Autodesk Inventor part; units mm, degrees
ref_plane "Work Plane1" through (36.2204, 0, -3.175) normal (1, 0, 0) x (0, 1, 0)
ref_plane "XZ Plane" through (0, 0, 0) normal (0, 1, 0) x (-1, 0, 0)
ref_plane "XY Plane" through (0, 0, 0) normal (0, 0, 1) x (1, 0, 0)
sketch "Sketch1" plane through (0, 0, 0) normal (0, 1, 0) x (-1, 0, 0)
  line L0 (-33.0454, 0) -> (0, 0)
  line L1 (0, 0) -> (0, 5.08)
  line L2 (0, 5.08) -> (3.175, 5.08)
  line L3 (-33.0454, 0) -> (-33.0454, -3.175)
  line L4 (-33.0454, -3.175) -> (-36.2204, -3.175)
  dimension "d1" = 33.0454
  dimension "d6" = 5.08
  dimension "d7" = 3.175
  dimension "d8" = 3.175
  dimension "d9" = 3.175
ref_plane "Work Plane1" through (36.2204, 0, -3.175) normal (1, 0, 0) x (0, 1, 0)
sketch "Sketch2" plane through (36.2204, 0, -3.175) normal (1, 0, 0) x (0, 1, 0)
  circle A0 centre (0, 0) radius 0.8
  point P0 (0, 3.175)
  dimension "d10" = 1.6
sweep "Sweep1" add profiles "Sketch2" path "Sketch1"
properties part number "foreDivePlanesLinkage" material "Stainless Steel"
Here's how the part is built. I have some questions about the finished solid (model axes, mm). A direction names the side the tool comes from. Give positions to 0.01 mm unless a question says otherwise; leave off trailing zeros. Write each loop counter-clockwise with the first axis right and the second up, starting at its lowest first coordinate (ties: lowest second). Pieces come first, ordered by that corner, then holes. Notation, with made-up numbers: (39.5, -38) -> (98.5, -38) arc R32 cw to (98.5, -5) -> close; hole circle Ø8 at (-21.5, 15). An arc over 180 degrees is marked (long way). Use one line per item in the form item = value.
1) If I drill on L1, parallel to X at y = 0.05, z = -2.5; L2, parallel to Z at x = 22.5, y = 0.1; L3, parallel to X at y = 0, z = -0.25, over which ranges is the centre line in solid material (lowest first)? Write a range as [from, to].
Verdict:
L1 = [32.25, 36.22]
L2 = [-0.79, 0.79]
L3 = [-0.8, 33.85]
2) I'm going to push a flat-ended pin straight in: pin 1 (2 mm diameter, centred on x = 6.5, z = -1, fed in from +Y). Where does the tip first touch, or does it pass through?
Verdict:
pin_1 = 0.8
3) On a 3-axis mill with a long thin cutter (end or side, diameter ignored), from which of +Z, -Z, +X, -X, +Y, -Y can I reach the whole of each face in a straight line? I mean faces 1 (the face through (16.28, -0.63, 0.49)), 2 (the face through (-1.66, -0.17, 5.86)), 3 (the face through (-3.175, 0, 5)), 4 (the face through (36.22, 0, -3)), 5 (the face through (34.65, -0.1, -3.97)). Say none if no direction works.
Verdict:
face_1 = none
face_2 = -X
face_3 = +Z, -Z, -X, +Y, -Y
face_4 = +Z, -Z, +X, +Y, -Y
face_5 = +X
4) Suppose I cut it at A-A (y = 0). Please give me the cut outline in (x, z) (3 decimals), and give its area (3 significant figures).
Verdict:
outline = (-3.175, 4.28) -> (-0.8, 4.28) -> (-0.8, -0.8) -> (32.245, -0.8) -> (32.245, -3.975) -> (36.22, -3.975) -> (36.22, -2.375) -> (33.845, -2.375) -> (33.845, 0.8) -> (0.8, 0.8) -> (0.8, 5.88) -> (-3.175, 5.88) -> close
area = 76.2 mm2
5) Suppose I cut it at B-B (z = 2). Please give me the cut outline in (x, y), and give its area (3 significant figures).
Verdict:
outline = circle Ø1.6 at (0, 0)
area = 2.01 mm2
6) Suppose I cut it at D-D (z = 5.08). Please give me the cut outline in (x, y) (3 decimals), and give its area (3 significant figures).
Verdict:
outline = (-3.175, -0.8) -> (0, -0.8) arc R0.8 ccw to (0, 0.8) -> (-3.175, 0.8) -> close
area = 6.09 mm2
